Design review of the part built by this model. Coordinates are the model's own, in mm. A direction names the side the tool comes from. Coordinates: 2 decimals unless noted, no trailing zeros. Write each loop counter-clockwise with the first axis right and the second up, starting at its lowest first coordinate (ties: lowest second). Pieces come first, ordered by that corner, then holes. Notation, with made-up numbers: (50.5, -34) - (75.5, -34) arc R16 ccw to (75.5, -14) - close; hole circle Ø9 at (8.25, -23.5). An arc over 180 degrees is marked (long way). Answer as CSV lines item,"result". Start each with the question number.
Q1. For line 1 along X through (y, z) = (-0.2, 27.5); line 2 along Z through (x, y) = (0.5, -1.55); line 3 along X through (y, z) = (-1.85, 202), list the stretches that pass through material, from the lowest coordinate up. Write a range as [from, to].
Q2. Mouldability with a two-part tool opening along Z and no side actions: class faces 6 (the face through (198.07, -1.97, 18.68)), 7 (the face through (-23.9, -1.97, 113.91)), 8 (the face through (-1, 0, 82)) as pulls with the +Z half, pulls with the -Z half, needs draft (parallel to the pull), parting line crosses it, or undercut.
Q3. We need section A-A (z = 47.5). Write out the cut boundary in (x, y).
Q4. Machinability: for faces 1 (the face through (2.16, -1.97, 161.47)), 2 (the face through (23.717, -1.972, 113.707)), 3 (the face through (-197.719, -1.972, 2.406)), 4 (the face through (-114.02, -1.97, 61.83)), 5 (the face through (94.01, -1.97, 47.1)), which of the approach directions +Z, -Z, +X, -X, +Y, -Y give a long, thin tool a straight path to every point of the face, cutting with its end or side? Answer none if there is none.
Q5. We need section B-B (x = 113). Write out the cut boundary in (y, z).
Q6. Clearance check with flat-ended pins moving along their axes: pin 1 (1.2 mm diameter, centred on x = 34, y = -3, fed in from +Z); pin 2 (2 mm diameter, centred on y = -2, z = 185.5, fed in from +X); pin 3 (2 mm diameter, centred on x = -134.5, y = -3, fed in from +Z). State where each tip first meets the part, or that it passes through.
Q7. We need section C-C (z = 138). Write out the cut boundary in (x, y), plus the area to 3 significant figures.
from build123d import *

# Parameters (mm, degrees)
F4_DEPTH = 4
F5_DEPTH = 25
F6_DEPTH = 4


with BuildPart() as f4:
    # F1 (on Front) → F4 (new body)
    with BuildSketch(Plane.XZ):
        with BuildLine():
            Line((-192, 0), (0, 0))
            Line((0, 0), (192, 0))
            ThreePointArc((192, 0), (197.656854, 2.343146), (200, 8))
            Line((200, 8), (200, 11.867938))
            ThreePointArc((200, 11.867938), (198.021286, 18.762229), (192.6875, 23.557777))
            Line((192.6875, 23.557777), (180.548051, 29.464027))
            ThreePointArc((180.548051, 29.464027), (179.402075, 29.533004), (178.542974, 28.77145))
            Line((178.542974, 28.77145), (177.667974, 26.973013))
            ThreePointArc((177.667974, 26.973013), (177.598997, 25.827036), (178.360551, 24.967935))
            Line((178.360551, 24.967935), (179.709379, 24.311685))
            ThreePointArc((179.709379, 24.311685), (180.724784, 23.166217), (180.632816, 21.638248))
            Line((180.632816, 21.638248), (179.101566, 18.490984))
            ThreePointArc((179.101566, 18.490984), (177.66973, 17.221727), (175.75977, 17.336688))
            Line((175.75977, 17.336688), (166.767586, 21.711688))
            ThreePointArc((166.767586, 21.711688), (165.498329, 23.143523), (165.61329, 25.053484))
            Line((165.61329, 25.053484), (169.11329, 32.247231))
            ThreePointArc((169.11329, 32.247231), (169.22825, 34.157192), (167.958994, 35.589027))
            Line((167.958994, 35.589027), (61.560664, 87.355393))
            ThreePointArc((61.560664, 87.355393), (56.583657, 90.555592), (52.498164, 94.835853))
            Line((52.498164, 94.835853), (43.525054, 106.8))
            ThreePointArc((43.525054, 106.8), (40.702763, 109.155418), (37.125054, 110))
            Line((37.125054, 110), (0, 110))
            Line((0, 110), (-37.125054, 110))
            ThreePointArc((-37.125054, 110), (-40.702763, 109.155418), (-43.525054, 106.8))
            Line((-43.525054, 106.8), (-52.498164, 94.835853))
            ThreePointArc((-52.498164, 94.835853), (-56.583657, 90.555592), (-61.560664, 87.355393))
            Line((-61.560664, 87.355393), (-167.958994, 35.589027))
            ThreePointArc((-167.958994, 35.589027), (-169.22825, 34.157192), (-169.11329, 32.247231))
            Line((-169.11329, 32.247231), (-165.61329, 25.053484))
            ThreePointArc((-165.61329, 25.053484), (-165.498329, 23.143523), (-166.767586, 21.711688))
            Line((-166.767586, 21.711688), (-175.75977, 17.336688))
            ThreePointArc((-175.75977, 17.336688), (-177.66973, 17.221727), (-179.101566, 18.490984))
            Line((-179.101566, 18.490984), (-180.632816, 21.638248))
            ThreePointArc((-180.632816, 21.638248), (-180.724784, 23.166217), (-179.709379, 24.311685))
            Line((-179.709379, 24.311685), (-178.360551, 24.967935))
            ThreePointArc((-178.360551, 24.967935), (-177.598997, 25.827036), (-177.667974, 26.973013))
            Line((-177.667974, 26.973013), (-178.542974, 28.77145))
            ThreePointArc((-178.542974, 28.77145), (-179.402075, 29.533004), (-180.548051, 29.464027))
            Line((-180.548051, 29.464027), (-192.6875, 23.557777))
            ThreePointArc((-192.6875, 23.557777), (-198.021286, 18.762229), (-200, 11.867938))
            Line((-200, 11.867938), (-200, 8))
            ThreePointArc((-200, 8), (-197.656854, 2.343146), (-192, 0))
        make_face()
    extrude(amount=F4_DEPTH)

    # F2 (on Front) → F5 (cut)
    with BuildSketch(Plane.XZ):
        with BuildLine():
            Line((-48.760248, 69.117535), (-138.003574, 25.697655))
            ThreePointArc((-138.003574, 25.697655), (-139.614511, 22.326563), (-136.691074, 20))
            Line((-136.691074, 20), (0, 20))
            Line((0, 20), (136.691074, 20))
            ThreePointArc((136.691074, 20), (139.614511, 22.326563), (138.003574, 25.697655))
            Line((138.003574, 25.697655), (48.760248, 69.117535))
            ThreePointArc((48.760248, 69.117535), (45.497375, 70.063317), (42.106154, 69.862174))
            ThreePointArc((42.106154, 69.862174), (21.192976, 66.219569), (0, 65))
            ThreePointArc((0, 65), (-21.192976, 66.219569), (-42.106154, 69.862174))
            ThreePointArc((-42.106154, 69.862174), (-45.497375, 70.063317), (-48.760248, 69.117535))
        make_face()
    extrude(amount=F5_DEPTH, mode=Mode.SUBTRACT)

    # F3 (on Front) → F6 (join)
    with BuildSketch(Plane.XZ):
        with BuildLine():
            ThreePointArc((32.807421, 110), (23.615033, 113.807612), (19.807421, 123))
            Line((19.807421, 123), (19.807421, 131))
            ThreePointArc((19.807421, 131), (21.789998, 138.891463), (27.266909, 144.908874))
            ThreePointArc((27.266909, 144.908874), (31.010618, 147.749106), (34.369203, 151.035771))
            ThreePointArc((34.369203, 151.035771), (39.024484, 158.627298), (40.648222, 167.383233))
            Line((40.648222, 167.383233), (40.648222, 191.518757))
            ThreePointArc((40.648222, 191.518757), (28.5597, 219.702824), (-0.19253, 230.369747))
            ThreePointArc((-0.19253, 230.369747), (-10.806946, 228.758492), (-20.884333, 225.056026))
            ThreePointArc((-20.884333, 225.056026), (-23.281736, 223.789035), (-25.589338, 222.365034))
            ThreePointArc((-25.589338, 222.365034), (-28.274915, 219.966), (-30.175497, 216.907327))
            ThreePointArc((-30.175497, 216.907327), (-33.010051, 207.223067), (-33.292141, 197.136441))
            ThreePointArc((-33.292141, 197.136441), (-29.36617, 192.336543), (-23.415442, 194.080419))
            ThreePointArc((-23.415442, 194.080419), (-20.197771, 198.205206), (-17.303473, 202.562993))
            ThreePointArc((-17.303473, 202.562993), (5.233861, 211.415378), (19.855876, 192.115305))
            Line((19.855876, 192.115305), (19.688146, 178.864043))
            ThreePointArc((19.688146, 178.864043), (17.438414, 171.2971), (11.551299, 166.037652))
            Line((11.551299, 166.037652), (-7.491809, 156.772539))
            ThreePointArc((-7.491809, 156.772539), (-9.889212, 155.505548), (-12.196814, 154.081547))
            ThreePointArc((-12.196814, 154.081547), (-14.846888, 151.724576), (-16.738336, 148.724473))
            ThreePointArc((-16.738336, 148.724473), (-19.325033, 140.813993), (-20.192579, 132.536671))
            Line((-20.192579, 132.536671), (-20.192579, 123))
            ThreePointArc((-20.192579, 123), (-24.000191, 113.807612), (-33.192579, 110))
            Line((-33.192579, 110), (32.807421, 110))
        make_face()
    extrude(amount=F6_DEPTH)


solid = f4.part
Results list:
1,line 1,"x = [-184.58, -177.92], [-166.8, -134.3], [134.3, 166.8], [177.92, 184.58]"
1,line 2,"z = [0, 20], [65, 160.66], [212.15, 230.4]"
1,line 3,"x = [-33.48, -17.65], [17.25, 39.21]"
2,face 6,"pulls with the +Z half"
2,face 7,"undercut"
2,face 8,"needs draft"
3,outline,"(-143.48, -4) - (-93.19, -4) - (-93.19, 0) - (-143.48, 0) - close; (93.19, -4) - (143.48, -4) - (143.48, 0) - (93.19, 0) - close"
4,face 1,"-X, +Y, -Y"
4,face 2,"+X, +Y, -Y"
4,face 3,"-Z, -X, +Y, -Y"
4,face 4,"+Z, -X, +Y, -Y"
4,face 5,"+Y, -Y"
5,outline,"(-4, 0) - (0, 0) - (0, 20) - (-4, 20) - close; (-4, 37.86) - (0, 37.86) - (0, 62.33) - (-4, 62.33) - close"
6,pin 1,"stops at z = 214.13"
6,pin 2,"stops at x = 40.65"
6,pin 3,"stops at z = 52.35"
7,outline,"(-19.82, -4) - (21.35, -4) - (21.35, 0) - (-19.82, 0) - close"
7,area,"165 mm2"
